Read the model definition and answer for the solid it produces. Units are mm, in the model's axes. Coordinates: 2 decimals unless noted, no trailing zeros. Write each loop counter-clockwise with the first axis right and the second up, starting at its lowest first coordinate (ties: lowest second). Pieces come first, ordered by that corner, then holes.
1) The part is cut by section A-A (z = 0). Determine the outline of the cut face in (x, y).
2) The part is cut by section B-B (x = 9.5). Determine the outline of the cut face in (y, z).
3) Each of these flat-tipped pins is pushed along its axis until it touches: pin 1 Ø10 at (y, z) = (211, 11.5) entering from -X; pin 2 Ø1.1 at (y, z) = (-359.5, 19.5) entering from -X; pin 3 Ø1.8 at (y, z) = (429.5, -18.5) entering from +X; pin 4 Ø8 at (x, y) = (-2, 9) entering from +Z. Where does it stop, or does it pass through?
4) Find the intervals of material crossed by line 1 (Y direction, x = -1, z = 18) (3 decimals); line 2 (X direction, y = 11, z = 2.5); line 3 (Z direction, x = 0, y = 230), in increasing order.
5) The part is cut by section D-D (y = -366). Determine the outline of the cut face in (x, z) (3 decimals), then the cut area to 3 significant figures.
6) Determine the mould class of faces 1 (the face through (-20.11, -6.76, -6.33)), 2 (the face through (3.8, 6.76, -17.11)), 3 (the face through (8, 482.6, 16)) for opening direction X: +X half, -X half, draft (parallel to the pull), parting line (faces both ways), or undercut.
7) The part is cut by section C-C (y = 133). Determine the outline of the cut face in (x, z).
Autodesk Inventor part; units mm, degrees
ref_plane "YZ Plane" through (0, 0, 0) normal (1, 0, 0) x (0, 1, 0)
ref_plane "XZ Plane" through (0, 0, 0) normal (0, 1, 0) x (-1, 0, 0)
ref_plane "XY Plane" through (0, 0, 0) normal (0, 0, 1) x (1, 0, 0)
sketch "Sketch1" plane through (0, 0, 0) normal (0, 1, 0) x (-1, 0, 0)
  circle A0 centre (0, 0) radius 21.082
  circle A1 centre (0, 0) radius 17.526
  dimension "d0" = 42.164
  dimension "d1" = 35.052
extrude "Extrusion1" add sketch "Sketch1" along normal mid plane 965.2
sketch "Sketch3" plane through (0, 0, 0) normal (0, 0, 1) x (1, 0, 0)
  line L0 (0, 474.6625) -> (0, 461.9625) construction
  line L1 (-3.175, 474.6625) -> (-3.175, 461.9625)
  line L2 (3.175, 461.9625) -> (3.175, 474.6625)
  arc A0 (3.175, 474.6625) -> (-3.175, 474.6625) centre (0, 474.6625) ccw
  arc A1 (-3.175, 461.9625) -> (3.175, 461.9625) centre (0, 461.9625) ccw
  line L3 (0, 436.5625) -> (0, 423.8625) construction
  line L4 (-3.175, 436.5625) -> (-3.175, 423.8625)
  line L5 (3.175, 423.8625) -> (3.175, 436.5625)
  arc A2 (3.175, 436.5625) -> (-3.175, 436.5625) centre (0, 436.5625) ccw
  arc A3 (-3.175, 423.8625) -> (3.175, 423.8625) centre (0, 423.8625) ccw
  line L6 (0, -298.45) -> (0, -450.85) construction
  line L7 (-3.175, -298.45) -> (-3.175, -450.85)
  line L8 (3.175, -450.85) -> (3.175, -298.45)
  arc A4 (3.175, -298.45) -> (-3.175, -298.45) centre (0, -298.45) ccw
  arc A5 (-3.175, -450.85) -> (3.175, -450.85) centre (0, -450.85) ccw
  line L9 (0, -450.85) -> (-6.35, -450.85) construction
  line L10 (0, -447.675) -> (-6.35, -447.675)
  line L11 (-6.35, -454.025) -> (0, -454.025)
  arc A6 (0, -454.025) -> (0, -447.675) centre (0, -450.85) ccw
  arc A7 (-6.35, -447.675) -> (-6.35, -454.025) centre (-6.35, -450.85) ccw
  line L12 (-21.082, -482.6) -> (21.082, -482.6)
  line L13 (21.082, 482.6) -> (-21.082, 482.6)
  point P0 (0, 468.3125)
  point P1 (0, 430.2125)
  point P2 (0, -374.65)
  point P3 (-3.175, -450.85)
  point P4 (0, -482.6)
  point P5 (-3.175, -447.675)
  dimension "d17" = 3.175
  dimension "d18" = 12.7
  dimension "d19" = 6.35
  dimension "d20" = 152.4
  dimension "d21" = 28.575
  dimension "d22" = 25.4
  dimension "d23" = 7.9375
extrude "Extrusion3" cut sketch "Sketch3" against normal through all contours A0 L2 A1 L1 | A2 L5 A3 L4
extrude "Extrusion4" cut sketch "Sketch3" along normal blind 25.4 contours A4 L8 A6 L10 L7 | L10 A6 A5 L7 | L7 A5 L11 A7 L10
properties part number "FE-120-007 Door Tube" material "Aluminum 6061"
Reported:
1. outline: (-21.08, -482.6) - (-17.53, -482.6) - (-17.53, 482.6) - (-21.08, 482.6) - close; (17.53, -482.6) - (21.08, -482.6) - (21.08, 482.6) - (17.53, 482.6) - close
2. outline: (-482.6, -18.82) - (482.6, -18.82) - (482.6, -14.73) - (-482.6, -14.73) - close; (-482.6, 14.73) - (482.6, 14.73) - (482.6, 18.82) - (-482.6, 18.82) - close
3. pin 1: stops at x = -20.05
3. pin 2: stops at x = -9.24
3. pin 3: stops at x = 11.61
3. pin 4: stops at z = 21.08
4. line 1: y = -482.6 to -454.025, -295.437 to 482.6
4. line 2: x = -20.93 to -17.35, 17.35 to 20.93
4. line 3: z = -21.08 to -17.53, 17.53 to 21.08
5. outline: (-3.175, 17.236) - (-3.175, 20.842) arc R21.082 ccw (long way) to (3.175, 20.842) - (3.175, 17.236) arc R17.526 cw (long way) to start
5. area: 409 mm2
6. face 1: parting line
6. face 2: undercut
6. face 3: draft
7. outline: circle Ø42.16 at (0, 0); hole circle Ø35.05 at (0, 0)
